Could you check a few things on this model? Use its own coordinates, in mm. Face numbers are marked on the shaded views. Coordinates: 2 decimals unless noted, no trailing zeros. Write each loop counter-clockwise with the first axis right and the second up, starting at its lowest first coordinate (ties: lowest second). Pieces come first, ordered by that corner, then holes.
```python
from build123d import *

# Parameters (mm, degrees)
F0_W     = 1270
F0_H     = 609.6
F1_DEPTH = 73.152
F2_T     = -2.667
F3_W     = 152.4
F3_H     = 101.6
F3_W_2   = 44.45
F3_H_2   = 25.4
F4_DEPTH = 73.153
F5_W     = 54.102
F5_H     = 7.874
F6_DEPTH = 7.874
F7_R     = 21.463
F8_DEPTH = 1270.001


with BuildPart() as f1:
    # F0 (on Top) → F1 (new body)
    with BuildSketch(Plane.XY):
        Rectangle(F0_W, F0_H)
    extrude(amount=F1_DEPTH)

    # F2
    f2_openings = [f1.faces().sort_by_distance(p)[0] for p in [
        (0, 0, 0),
    ]]
    offset(amount=F2_T, openings=f2_openings)

    # F3 (on face) → F4 (cut, through all)
    with BuildSketch(Plane.XY.offset(73.152)):
        with Locations((-457.2, 228.6)):
            Rectangle(F3_W, F3_H)
        Polygon((-434.975, 127), (-381, 177.8), (-533.4, 177.8), (-479.425, 127), align=None)
        with Locations((-457.2, 114.3)):
            Rectangle(F3_W_2, F3_H_2)
        with Locations((-279.4, -152.4)):
            Rectangle(F3_W, F3_H)
        Polygon((-355.6, -203.2), (-301.625, -254), (-257.175, -254), (-203.2, -203.2), align=None)
        with Locations((-279.4, -266.7)):
            Rectangle(F3_W_2, F3_H_2)
        with Locations((279.4, -266.7)):
            Rectangle(F3_W_2, F3_H_2)
        with Locations((279.4, -152.4)):
            Rectangle(F3_W, F3_H)
        with Locations((457.2, 114.3)):
            Rectangle(F3_W_2, F3_H_2)
        Polygon((381, 177.8), (434.975, 127), (479.425, 127), (533.4, 177.8), align=None)
        with Locations((457.2, 228.6)):
            Rectangle(F3_W, F3_H)
        Polygon((203.2, -203.2), (257.175, -254), (301.625, -254), (355.6, -203.2), align=None)
    extrude(amount=-F4_DEPTH, mode=Mode.SUBTRACT)

    # F5 (on face) → F6 (cut)
    with BuildSketch(Plane.XY.offset(73.152)):
        with Locations((-607.949, 300.863)):
            Rectangle(F5_W, F5_H)
        with Locations((-200.025, 300.863)):
            Rectangle(F5_W, F5_H)
        with Locations((200.025, 300.863)):
            Rectangle(F5_W, F5_H)
        with Locations((607.949, 300.863)):
            Rectangle(F5_W, F5_H)
        with Locations((607.949, -300.863)):
            Rectangle(F5_W, F5_H)
        with Locations((200.025, -300.863)):
            Rectangle(F5_W, F5_H)
        with Locations((-200.025, -300.863)):
            Rectangle(F5_W, F5_H)
        with Locations((-607.949, -300.863)):
            Rectangle(F5_W, F5_H)
    extrude(amount=-F6_DEPTH, mode=Mode.SUBTRACT)

    # F7 (on face) → F8 (cut, through all)
    with BuildSketch(Plane.YZ.offset(635)):
        with Locations((223.266, 35.052)):
            Circle(F7_R)
        with Locations((-223.266, 35.052)):
            Circle(F7_R)
    extrude(amount=-F8_DEPTH, mode=Mode.SUBTRACT)


solid = f1.part
```
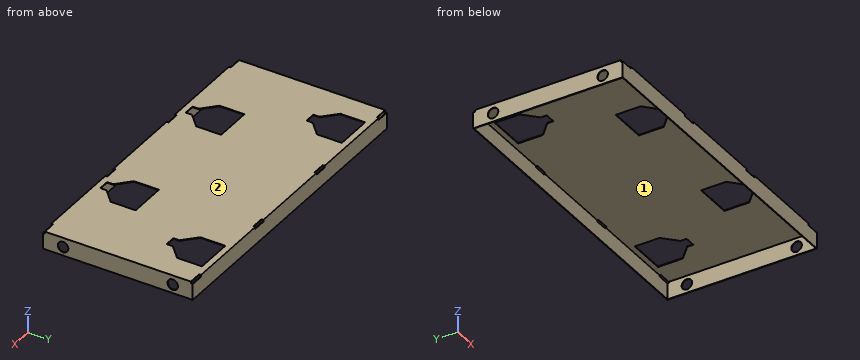
1. Please list where these lines run through material, in increasing order: line 1 along X through (y, z) = (15, 44.5); line 2 along Y through (x, z) = (-388, 65.5); line 3 along Z through (x, y) = (-89, -196) (3 decimals).
Verdict:
line 1: x = -635 to -632.33, 632.33 to 635
line 2: y = -304.8 to -302.13, 302.13 to 304.8
line 3: z = 70.485 to 73.152
2. I want a section at B-B on x = -315. Please give me the cut outline in (y, z) (3 decimals), plus the area to 3 significant figures.
Verdict:
outline: (-304.8, 0) - (-302.133, 0) - (-302.133, 70.485) - (-241.412, 70.485) - (-241.412, 73.152) - (-304.8, 73.152) - close; (-101.6, 70.485) - (302.133, 70.485) - (302.133, 0) - (304.8, 0) - (304.8, 73.152) - (-101.6, 73.152) - close
area: 1,630 mm2
3. I want a section at C-C on y = 11. Please give me the cut outline in (x, z) (3 decimals), plus the area to 3 significant figures.
Verdict:
outline: (-635, 0) - (-632.333, 0) - (-632.333, 70.485) - (632.333, 70.485) - (632.333, 0) - (635, 0) - (635, 73.152) - (-635, 73.152) - close
area: 3,760 mm2
4. For pin 1 (6.5 mm diameter, centred on x = -600.5, y = -302.5, fed in from +Z); pin 2 (2 mm diameter, centred on x = 210, z = 72.5, fed in from -Y); pin 3 (12 mm diameter, centred on x = 190, y = -146.5, fed in from -Z) (3 decimals), each with a flat end and sliding along its axis, tell me the tip position at first contact or that it passes through.
Verdict:
pin 1: stops at z = 65.28
pin 2: stops at y = -296.93
pin 3: stops at z = 70.485
5. If we mould it in two halves opening along Y, with no side actions, what happens to the marked faces 1 and 2? For each: pulls with the +Y half, pulls with the -Y half, needs draft (parallel to the pull), parting line crosses it, or undercut.
Verdict:
face 1: undercut
face 2: needs draft
6. I want a section at A-A on y = 113. Please give me the cut outline in (x, z) (3 decimals), plus the area to 3 significant figures.
Verdict:
outline: (-635, 0) - (-632.333, 0) - (-632.333, 70.485) - (-479.425, 70.485) - (-479.425, 73.152) - (-635, 73.152) - close; (-434.975, 70.485) - (434.975, 70.485) - (434.975, 73.152) - (-434.975, 73.152) - close; (479.425, 70.485) - (632.333, 70.485) - (632.333, 0) - (635, 0) - (635, 73.152) - (479.425, 73.152) - close
area: 3,530 mm2
7. I want a section at D-D on x = 118.5. Please give me the cut outline in (y, z) (3 decimals).
Verdict:
outline: (-304.8, 0) - (-302.133, 0) - (-302.133, 70.485) - (302.133, 70.485) - (302.133, 0) - (304.8, 0) - (304.8, 73.152) - (-304.8, 73.152) - close
